Input: dimensioned drawing with shaded views. Units: mm. Origin: part minimum x, y, z. A direction names the side the tool comes from. Round coordinates to 2 decimals unless told otherwise and drop trailing zeros. Loops run counter-clockwise (first coordinate to the right, second up) from the corner with the lowest first, then second, coordinate; pieces in that order, holes last. Notation, with made-up numbers: M 14,3.25 L 40,3.25 A23 ccw 40,19.25 Z; hole C 5.5,-38.5 d8. An arc over 180 degrees is marked long. Return JSON: item names as keys, results as strings.
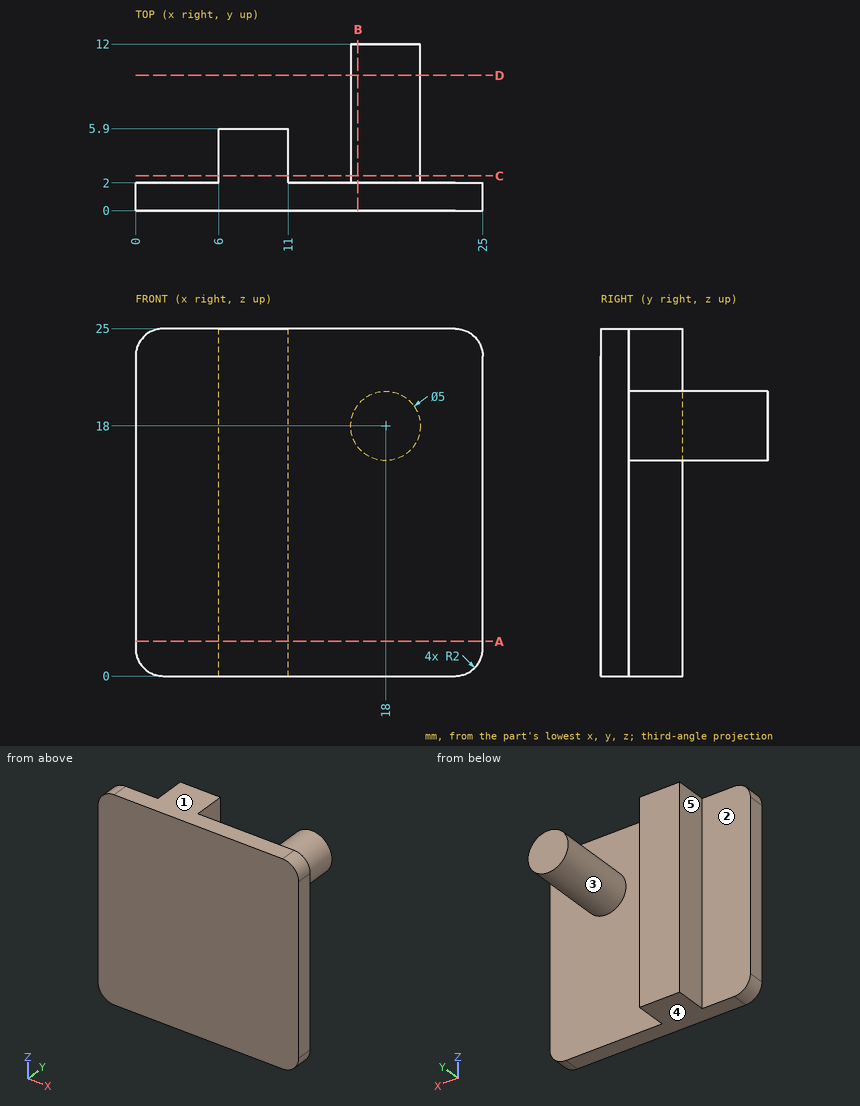
Q1. Pin query (flat end, axial travel): pin 1 (4.5 mm diameter, centred on y = 5, z = 16, fed in from +X); pin 2 (2 mm diameter, centred on y = 4.5, z = 13, fed in from -X); pin 3 (1.5 mm diameter, centred on y = 10, z = 16, fed in from +X). Return the tip coordinate at first contact, or that it passes through.
Determined:
{"pin 1": "stops at x = 20.5", "pin 2": "stops at x = 6", "pin 3": "stops at x = 20.17"}
Q2. Section query C-C (y = 2.5). Output: boundary loops of the cut face in (x, z), plus the area to 3 significant figures.
Determined:
{"outline": "M 6,0 L 11,0 L 11,25 L 6,25 Z; C 18,18 d5", "area": "145 mm^2"}
Q3. Section query D-D (y = 9.75). Output: boundary loops of the cut face in (x, z).
Determined:
{"outline": "C 18,18 d5"}
Q4. Section query A-A (z = 2.5). Output: boundary loops of the cut face in (x, y).
Determined:
{"outline": "M 0,0 L 25,0 L 25,2 L 11,2 L 11,5.9 L 6,5.9 L 6,2 L 0,2 Z"}
Q5. Pull-direction query (X, two-part tool) for the marked faces 3, 4 and 5; classes: pulls with the +X half, pulls with the -X half, needs draft (parallel to the pull), parting line crosses it, or undercut.
Determined:
{"face 3": "undercut", "face 4": "needs draft", "face 5": "pulls with the -X half"}
Q6. Material intervals for L1, parallel to Y at x = 3, z = 12.25; L2, parallel to Y at x = 7.25, z = 14; L3, parallel to X at y = 5.25, z = 11, sorted ascending.
Determined:
{"L1": "y = 0 to 2", "L2": "y = 0 to 5.9", "L3": "x = 6 to 11"}
Q7. Section query B-B (x = 16). Output: boundary loops of the cut face in (y, z), plus the area to 3 significant figures.
Determined:
{"outline": "M 0,0 L 2,0 L 2,16.5 L 12,16.5 L 12,19.5 L 2,19.5 L 2,25 L 0,25 Z", "area": "80.0 mm^2"}
Q8. Reachability of the marked faces 1 and 2 from +Z, -Z, +X, -X, +Y, -Y: full face, straight path, thin tool, end or side. Return the list, or none.
Determined:
{"face 1": "+Z, +X, -X, +Y, -Y", "face 2": "+Z, -Z, -X, +Y"}
